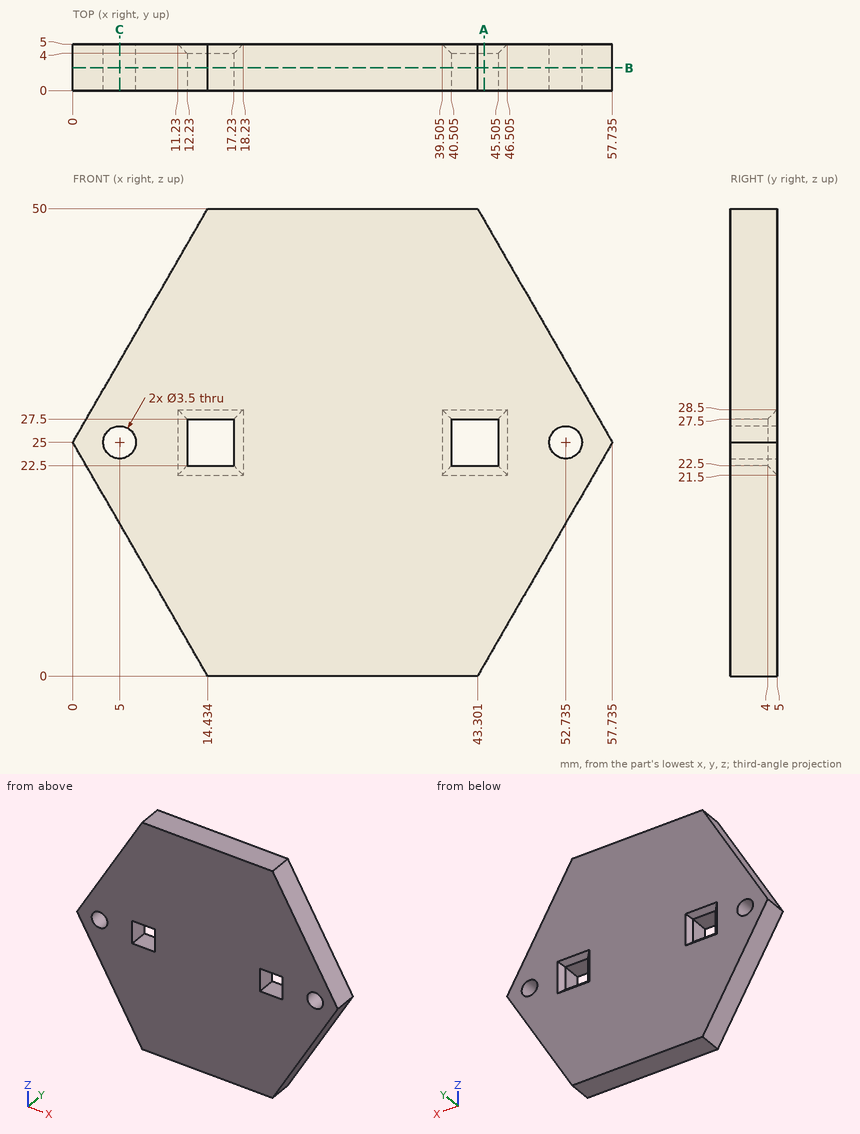
Input: dimensioned drawing with shaded views. Units: mm. Origin: part minimum x, y, z. Round coordinates to 2 decimals unless told otherwise and drop trailing zeros. Order: outer loops, then holes, each group sorted by start corner. A loop starts at its lowest first (then second) coordinate and runs counter-clockwise, first axis right, second up. Notation, with made-up numbers: (11, -13) - (64, -13) arc R30 cw to (64, 11) - close; hole circle Ø10 at (20, 14.5). An arc over 180 degrees is marked (long way). Write item = value, one per line. Start each with the question number.
Q1. Pin query (flat end, axial travel): pin 1 (2 mm diameter, centred on x = 52.74, z = 25, fed in from +Y); pin 2 (2 mm diameter, centred on x = 52, y = 2, fed in from +Z) (1 decimal); pin 3 (1.5 mm diameter, centred on y = 1.5, z = 43.5, fed in from -X). Return the tip coordinate at first contact, or that it passes through.
Q2. Cut plane C-C on x = 5. Return the cut outline in (y, z).
Q3. Cut plane A-A on x = 44. Return the cut outline in (y, z).
Q4. Ray query, line 1 (Z direction, x = 6.5, y = 2.8); line 2 (Z direction, x = 8, y = 1.2) (1 decimal); line 3 (X direction, y = 2.3, z = 13). Return the intervals inside material, ascending. Write a range as from..to.
Q5. Cut plane B-B on y = 2.45. Give the number of separate pieces and of enclosed holes in the cut face, and give its area (3 significant figures).
Outcome:
q1.pin_1 = through
q1.pin_2 = 36.7
q1.pin_3 = 10.25
q2.outline = (0, 16.34) - (5, 16.34) - (5, 23.25) - (0, 23.25) - close; (0, 26.75) - (5, 26.75) - (5, 33.66) - (0, 33.66) - close
q3.outline = (0, 1.21) - (5, 1.21) - (5, 21.5) - (4, 22.5) - (0, 22.5) - close; (0, 27.5) - (4, 27.5) - (5, 28.5) - (5, 48.79) - (0, 48.79) - close
q4.line_1 = 13.74..24.1, 25.9..36.26
q4.line_2 = 11.1..38.9
q4.line_3 = 6.93..50.81
q5.separate_pieces = 1
q5.enclosed_holes = 4
q5.area = 2,100 mm^2
